The listing builds one solid part. Answer for the finished solid, in the listing's coordinates (mm). A direction names the side the tool comes from. Coordinates: 2 decimals unless noted, no trailing zeros. Order: outer loops, then holes, each group sorted by start corner. A loop starts at its lowest first (then second) coordinate and runs counter-clockwise, first axis right, second up. Notation, with made-up numbers: (29.25, 66.5) -> (64.25, 66.5) arc R23 ccw to (64.25, 76.5) -> close; hole circle Ø6 at (33, 83.25). An arc over 180 degrees is marked (long way). Answer in a Markdown table with one row per item. Add a question column.
```python
from build123d import *
from build123d.topology import SkipClean

# Parameters (mm, degrees)
BOSS_EXTRU_1_DEPTH      = 5
BOSS_EXTRU_3_START      = 2
BOSS_EXTRU_3_DEPTH      = 2
ESQUISSE5_R             = 0.5
ESQUISSE5_R_2           = 2.5
ENL_V_MAT_EXTRU_1_DEPTH = 2
ESQUISSE7_R             = 2.5
ENL_V_MAT_EXTRU_2_DEPTH = 24.906066176


with BuildPart() as part:
    # Esquisse1 → Boss.-Extru.1 (new body)
    with BuildSketch(Plane.XY):
        with BuildLine():
            Line((-1.732050808, 1), (1.732050808, 1))
            ThreePointArc((1.732050808, 1), (1.931851653, 0.51763809), (2, 0))
            Line((2, 0), (17.5, 0))
            ThreePointArc((17.5, 0), (0, 17.5), (-17.5, 0))
            Line((-17.5, 0), (-2, 0))
            ThreePointArc((-2, 0), (-1.931851653, 0.51763809), (-1.732050808, 1))
        make_face()
    extrude(amount=BOSS_EXTRU_1_DEPTH)

    # Esquisse3 → Boss.-Extru.3 (add)
    with SkipClean():  # the faces are left unmerged after this step: merging them gives an invalid solid
        with BuildSketch(Plane(origin=(0, 0, 0), x_dir=(-1, 0, 0), z_dir=(0, 0, -1)).offset(BOSS_EXTRU_3_START)):
            with BuildLine():
                Line((0, 2), (0, 17.5))
                ThreePointArc((0, 17.5), (-12.374368671, 12.374368671), (-17.5, 0))
                Line((-17.5, 0), (-2, 0))
                ThreePointArc((-2, 0), (-1.931851653, 0.51763809), (-1.732050808, 1))
                ThreePointArc((-1.732050808, 1), (-1, 1.732050808), (0, 2))
            make_face()
            with BuildLine():
                ThreePointArc((17.5, 0), (12.374368671, 12.374368671), (0, 17.5))
                Line((0, 17.5), (0, 2))
                ThreePointArc((0, 2), (1, 1.732050808), (1.732050808, 1))
                ThreePointArc((1.732050808, 1), (1.931851653, 0.51763809), (2, 0))
                Line((2, 0), (17.5, 0))
            make_face()
        extrude(amount=-BOSS_EXTRU_3_DEPTH)

    # Esquisse5 → Enlèv. mat.-Extru.1 (cut)
    with SkipClean():  # the faces are left unmerged after this step: merging them gives an invalid solid
        with BuildSketch(Plane.XZ):
            with Locations(Location((-10.5, 1.5, 0), (0, 0, 270))):
                Circle(ESQUISSE5_R)
            with Locations(Location((10.5, 1.5, 0), (0, 0, 270))):
                Circle(ESQUISSE5_R_2)
        extrude(amount=-ENL_V_MAT_EXTRU_1_DEPTH, mode=Mode.SUBTRACT)

    # Esquisse7 → Enlèv. mat.-Extru.2 (cut, through all)
    with SkipClean():  # the faces are left unmerged after this step: merging them gives an invalid solid
        with BuildSketch(Plane.XZ.offset(-2)):
            with Locations(Location((10.5, 1.5, 0), (0, 0, 270))):
                Circle(ESQUISSE7_R)
        extrude(amount=-ENL_V_MAT_EXTRU_2_DEPTH, mode=Mode.SUBTRACT)


solid = part.part
```
Q1. For faces 1 (the face through (0, 7, 5)), 2 (the face through (-10.5, 2, 1.5)), 3 (the face through (0, 1.4, 0)), determine the directions among +Z, -Z, +X, -X, +Y, -Y from which every point of the face is accessible in a straight line to the end or side of a thin tool.
Q2. Determine the mould class of faces 4 (the face through (-10.988, 0.986, 1.608)), 5 (the face through (0, 7, -2)), 6 (the face through (0, 1, 2)) for opening direction Z: +Z half, -Z half, draft (parallel to the pull), parting line (faces both ways), or undercut.
Q3. A cutting plane is placed at B-B (x = -10.5). Determine the outline of the cut face in (y, z).
Q4. A cutting plane is placed at D-D (y = 4.5). Determine the outline of the cut face in (x, z), then the cut area to 3 significant figures.
Q5. Straight lines are drawn through the part: line 1 (Z direction, x = 10.5, y = 8.75); line 2 (X direction, y = 1.5, z = 1.5); line 3 (X direction, y = 10.75, z = 2). For each, find the intervals that lie inside material, in ascending order.
Q6. Given pin 1 (1.1 mm diameter, centred on x = -10.5, z = 1.5, fed in from -Y); pin 2 (1.5 mm diameter, centred on x = -5.5, z = 3.5, fed in from +Y); pin 3 (1 mm diameter, centred on y = 5.5, z = -0.5, fed in from +X); pin 4 (3 mm diameter, centred on y = 4.5, z = -1, fed in from +X), each flat-ended and moving along its own axis, determine where each tip first touches the part or whether it passes through.
Q7. A cutting plane is placed at A-A (x = 10.5). Determine the outline of the cut face in (y, z), then the cut area to 3 significant figures.
Q8. A cutting plane is placed at C-C (z = 1.5). Determine the outline of the cut face in (x, y), then the cut area to 3 significant figures.
Returned:
| question | item | result |
|---|---|---|
| 1 | face 1 | +Z, +X, -X, +Y, -Y |
| 1 | face 2 | -Y |
| 1 | face 3 | -Z, -Y |
| 2 | face 4 | undercut |
| 2 | face 5 | -Z half |
| 2 | face 6 | draft |
| 3 | outline | (0, -2) -> (14, -2) -> (14, 5) -> (0, 5) -> (0, 2) -> (2, 2) -> (2, 1) -> (0, 1) -> close |
| 4 | outline | (-16.91, -2) -> (16.91, -2) -> (16.91, 5) -> (-16.91, 5) -> close; hole circle Ø5 at (10.5, 1.5) |
| 4 | area | 217 mm² |
| 5 | line 1 | z = -2 to -1, 4 to 5 |
| 5 | line 2 | x = -17.44 to -11, -10 to 8, 13 to 17.44 |
| 5 | line 3 | x = -13.81 to 8.05, 12.95 to 13.81 |
| 6 | pin 1 | stops at y = 0 |
| 6 | pin 2 | stops at y = 16.84 |
| 6 | pin 3 | stops at x = 16.77 |
| 6 | pin 4 | stops at x = 17.24 |
| 7 | outline | (0, -2) -> (14, -2) -> (14, -1) -> (0, -1) -> close; (0, 4) -> (14, 4) -> (14, 5) -> (0, 5) -> close |
| 7 | area | 28.0 mm² |
| 8 | outline | (-17.5, 0) -> (-11, 0) -> (-11, 2) -> (-10, 2) -> (-10, 0) -> (-2, 0) arc R2 cw to (-1.73, 1) -> (1.73, 1) arc R2 cw to (2, 0) -> (8, 0) -> (8, 15.56) arc R17.5 ccw to start; (13, 0) -> (17.5, 0) arc R17.5 ccw to (13, 11.72) -> close |
| 8 | area | 406 mm² |
